Check sheet for the modelled part. Datum: model origin and axes. Units: mm. A direction names the side the tool comes from. Round coordinates to 2 decimals unless told otherwise and drop trailing zeros. Order: outer loops, then holes, each group sorted by start corner. A loop starts at its lowest first (then second) coordinate and runs counter-clockwise, first axis right, second up. Notation, with made-up numbers: (7.25, -23.75) -> (26.25, -23.75) arc R25 cw to (26.25, 10.25) -> close; hole circle Ø8 at (-24.75, -8). An arc over 180 degrees is marked (long way). Answer in a Markdown table with one row per item. Add a question column.
1. Draft check along Y on faces 1 (the cylindrical face through (-2.688, 66.716, -110.07)), 2 (the flat face through (25, 75, -110)), 3 (the flat face through (25, -75, -110)), 4 (the flat face through (100, 0, -110)). Enter one of: +Y half, -Y half, draft (parallel to the pull), parting line (faces both ways), or undercut.
2. Access from +Z, -Z, +X, -X, +Y, -Y to the whole of each face (thin tool, end or side, straight path). Record for faces 5 (the cylindrical face through (-74.98, 1.65, -109.93)), 6 (the cylindrical face through (47.69, 15.02, 1.47)).
3. Depth check by flat-ended pin: P1, Ø1, axis at y = -33, z = -79.5, coming from the +X side; P2, Ø6, axis at x = -48.5, z = -14, coming from the +Y side; P3, Ø10, axis at x = -13.5, z = -22.5, coming from the +Y side. Enter the tip coordinate at first touch or a pass-through.
4. Material ranges on L1, parallel to Y at x = 0, z = -111.25; L2, parallel to Z at x = 59, y = -67; L3, parallel to Y at x = -62.5, z = -109.5, recorded low to high. Write a range as from..to.
5. Sectioned sample at A-A, the plane y = 0. Record the boundary of the cut face in (x, z).
6. Sectioned sample at B-B, the plane x = 34.5. Record the boundary of the cut face in (y, z).
7. Sectioned sample at D-D, the plane y = -38. Record the boundary of the cut face in (x, z), then the cut area to 3 significant figures.
8. Sectioned sample at C-C, the plane z = 74.5. Record the boundary of the cut face in (x, y), then the cut area to 3 significant figures.
```python
from build123d import *

# Parameters (mm, degrees)
SKETCH1_R           = 50
BOSS_EXTRUDE1_DEPTH = 105
BOSS_EXTRUDE2_DEPTH = 10
SKETCH3_R           = 5
CUT_EXTRUDE1_DEPTH  = 10
FILLET1_R           = 50


with BuildPart() as part:
    # Sketch1 → Boss-Extrude1 (new, symmetric)
    with BuildSketch(Plane.XY):
        Circle(SKETCH1_R)
    extrude(amount=BOSS_EXTRUDE1_DEPTH, both=True)

    # Sketch2 → Boss-Extrude2 (add)
    with BuildSketch(Plane(origin=(0, 0, -105), x_dir=(-1, 0, 0), z_dir=(0, 0, -1))):
        with BuildLine():
            Line((0, -75), (-100, -75))
            Line((-100, -75), (-100, 75))
            Line((-100, 75), (0, 75))
            ThreePointArc((0, 75), (75, 0), (0, -75))
        make_face()
    extrude(amount=BOSS_EXTRUDE2_DEPTH)

    # Sketch3 → Cut-Extrude1 (cut)
    with BuildSketch(Plane(origin=(0, 0, -115), x_dir=(-1, 0, 0), z_dir=(0, 0, -1))):
        with Locations((0, 62.5)):
            Circle(SKETCH3_R)
        with Locations((0, -62.5)):
            Circle(SKETCH3_R)
        with Locations((62.5, 0)):
            Circle(SKETCH3_R)
    extrude(amount=-CUT_EXTRUDE1_DEPTH, mode=Mode.SUBTRACT)

    # Fillet1
    fillet1_edges = [part.edges().sort_by_distance(p)[0] for p in [
        (100, 75, -110),
        (100, -75, -110),
    ]]
    fillet(fillet1_edges, radius=FILLET1_R)


solid = part.part
```
Answer key:
| question | item | result |
|---|---|---|
| 1 | face 1 | undercut |
| 1 | face 2 | +Y half |
| 1 | face 3 | -Y half |
| 1 | face 4 | draft |
| 2 | face 5 | +Z, -Z, -X |
| 2 | face 6 | +Z |
| 3 | P1 | stops at x = 38 |
| 3 | P2 | stops at y = 20.73 |
| 3 | P3 | stops at y = 49.27 |
| 4 | L1 | y = -75..-67.5, -57.5..57.5, 67.5..75 |
| 4 | L2 | z = -115..-105 |
| 4 | L3 | y = -41.46..-5, 5..41.46 |
| 5 | outline | (-75, -115) -> (-67.5, -115) -> (-67.5, -105) -> (-75, -105) -> close; (-57.5, -115) -> (100, -115) -> (100, -105) -> (50, -105) -> (50, 105) -> (-50, 105) -> (-50, -105) -> (-57.5, -105) -> close |
| 6 | outline | (-75, -115) -> (75, -115) -> (75, -105) -> (36.19, -105) -> (36.19, 105) -> (-36.19, 105) -> (-36.19, -105) -> (-75, -105) -> close |
| 7 | outline | (-64.66, -115) -> (98.28, -115) -> (98.28, -105) -> (32.5, -105) -> (32.5, 105) -> (-32.5, 105) -> (-32.5, -105) -> (-64.66, -105) -> close |
| 7 | area | 15,300 mm² |
| 8 | outline | circle Ø100 at (0, 0) |
| 8 | area | 7,850 mm² |
